For this review, take the finished solid that the model builds, in its own axes (mm). Face numbers are marked on the shaded views. A direction names the side the tool comes from. Give positions to 0.01 mm unless a question says otherwise; leave off trailing zeros. Order: outer loops, then holes, each group sorted by start corner. A loop starts at its lowest first (then second) coordinate and runs counter-clockwise, first axis right, second up. Notation, with made-up numbers: (14, 58) - (40, 58) arc R14 ccw to (40, 62) - close; hole circle Ø7 at (19.5, -23). An arc over 180 degrees is marked (long way). One line per item, written item: value.
Autodesk Inventor part; units mm, degrees
ref_plane "YZ Plane" through (0, 0, 0) normal (1, 0, 0) x (0, 1, 0)
ref_plane "XZ Plane" through (0, 0, 0) normal (0, 1, 0) x (-1, 0, 0)
ref_plane "XY Plane" through (0, 0, 0) normal (0, 0, 1) x (1, 0, 0)
sketch "Sketch1" plane through (0, 0, 0) normal (0, 0, 1) x (1, 0, 0)
  line L0 (0, 0) -> (25, 0)
  line L1 (25, 0) -> (25, 40)
  line L2 (25, 40) -> (0, 40)
  line L3 (0, 40) -> (0, 0)
  dimension "d1" = 25
  dimension "d2" = 40
  dimension "d3" = 25
extrude "Extrusion1" add sketch "Sketch1" against normal blind 30
sketch "Sketch2" plane through (25, 0, 0) normal (1, 0, 0) x (0, 0, -1)
  line L0 (0, 0) -> (30, 0)
  circle A0 centre (15, 6.56) radius 2.46
extrude "Extrusion2" cut sketch "Sketch2" against normal blind 30
sketch "Sketch3" plane through (0, 0, 0) normal (-1, 0, 0) x (0, 0, 1)
  line L0 (0, 0) -> (-30, 0)
  line L1 (-25.05, 0) -> (-4.95, 0)
  line L2 (-4.95, 0) -> (-4.95, 33.12)
  line L3 (-4.95, 33.12) -> (-25.05, 33.12)
  line L4 (-25.05, 33.12) -> (-25.05, 0)
  dimension "d11" = 20.1
extrude "Extrusion3" cut sketch "Sketch3" against normal blind 20
sketch "Sketch4" plane through (0, 0, 0) normal (0, -1, 0) x (1, 0, 0)
  line L0 (20, -4.95) -> (20, -25.05)
  line L1 (20, -15) -> (25, -15)
  line L2 (25, 0) -> (25, -30)
  line L3 (20, -8.025) -> (25, -8.025)
  line L4 (25, -8.025) -> (25, -21.975)
  line L5 (25, -21.975) -> (20, -21.975)
  line L6 (20, -21.975) -> (20, -8.025)
  line L7 (20, -8.025) -> (25, -21.975) construction
  line L8 (25, -8.025) -> (20, -21.975) construction
  line L9 (25, -12.54) -> (25, -17.46)
  point P0 (0, 0)
  point P1 (22.5, -15)
  dimension "d14" = 13.95
extrude "Extrusion4" add sketch "Sketch4" along normal blind 15
sketch "Sketch5" plane through (20, 0, 0) normal (-1, 0, 0) x (0, 0, 1)
  circle A0 centre (-15, 6.56) radius 2.46
  circle A1 centre (-15, 6.56) radius 4.7025
  circle A2 centre (-15, 6.56) radius 2.46
  circle A3 centre (-15, 6.56) radius 2.46
  point P0 (0, 0)
  dimension "d17" = 9.405
extrude "Extrusion5" cut sketch "Sketch5" against normal blind 2.1
sketch "Sketch6" plane through (25, 0, 0) normal (1, 0, 0) x (0, 0, -1)
  circle A0 centre (15, 6.56) radius 4.7025
  line L0 (15, 6.56) -> (15, 23.56)
  circle A1 centre (15, 23.56) radius 2.46
  point P0 (0, 0)
  dimension "d20" = 17
  dimension "d21" = 4.92
extrude "Extrusion6" cut sketch "Sketch6" against normal blind 10 contours A1
sketch "Sketch7" plane through (20, 0, 0) normal (-1, 0, 0) x (0, 0, 1)
  circle A0 centre (-15, 23.56) radius 2.46
  circle A1 centre (-15, 23.56) radius 4.7025
  point P0 (0, 0)
  dimension "d24" = 9.405
extrude "Extrusion7" cut sketch "Sketch7" against normal blind 2.1
sketch "Sketch9" plane through (25, 0, 0) normal (1, 0, 0) x (0, 0, -1)
  circle A0 centre (15, 6.56) radius 2.46
  circle A1 centre (15, 6.56) radius 2.46
  circle A2 centre (15, 23.56) radius 2.46
  circle A3 centre (15, 23.56) radius 2.46
  line L0 (30, 40) -> (30, 0)
  line L1 (30, 0) -> (30, 40)
  line L2 (30, 40) -> (0, 40)
  line L3 (0, 40) -> (0, 0)
  line L4 (0, 0) -> (8.025, 0)
  line L5 (21.975, 0) -> (21.975, -15)
  line L6 (21.975, -15) -> (8.025, -15)
  line L7 (8.025, -15) -> (8.025, 0)
  line L8 (0, 0) -> (8.025, 0)
  line L9 (21.975, 0) -> (30, 0)
extrude "Extrusion8" add sketch "Sketch9" along normal blind 5
sketch "Sketch10" plane through (0, 40, 0) normal (0, 1, 0) x (1, 0, 0)
  line L0 (0, 30) -> (30, 30)
  line L1 (30, 0) -> (0, 0)
  line L2 (0, 30) -> (30, 30)
  line L3 (30, 30) -> (30, 0)
  line L4 (30, 0) -> (0, 0)
  line L5 (0, 0) -> (0, 30)
extrude "Extrusion9" add sketch "Sketch10" along normal blind 30
sketch "Sketch12" plane through (30, 0, 0) normal (1, 0, 0) x (0, 0, -1)
  circle A0 centre (15, 6.56) radius 2.46
  line L0 (15, 6.56) -> (15, 15.06)
  circle A1 centre (15, 15.06) radius 2.525
  point P0 (0, 0)
  dimension "d31" = 8.5
  dimension "d33" = 5.05
extrude "Extrusion10" cut sketch "Sketch12" against normal blind 30 contours A1
sketch "Sketch14" plane through (0, 0, 0) normal (0, 0, 1) x (1, 0, 0)
  line L0 (30, 70) -> (0, 70)
  line L1 (0, 70) -> (0, 85)
  line L2 (-15, 100) -> (-23, 100)
  line L3 (30, 0) -> (30, 70)
  line L4 (30, 113) -> (30, 70)
  arc A0 (0, 85) -> (-15, 100) centre (-15, 85) ccw
  line L5 (30, 105) -> (30, 100)
  line L6 (-23, 128) -> (15, 128)
  line L7 (30, 113) -> (15, 128)
  line L8 (-23, 128) -> (-23, 100)
  point P0 (0, 0)
  point P1 (0, 100)
  dimension "d47" = 30
  dimension "d54" = 15
  dimension "d69" = 28
extrude "Extrusion12" add sketch "Sketch14" against normal blind 30
sketch "Sketch15" plane through (0, 0, -25.05) normal (-1, 0, 0) x (0, 0, 1)
  line L0 (0, 33.12) -> (20.1, 33.12)
  line L1 (20.1, 33.12) -> (20.1, 0)
  line L2 (0, 33.12) -> (20.1, 33.12)
  line L3 (20.1, 33.12) -> (20.1, 31.1)
  line L4 (20.1, 31.1) -> (0, 31.1)
  line L5 (0, 31.1) -> (0, 33.12)
  point P0 (25.05, 0)
  dimension "d57" = 2.02
extrude "Extrusion13" add sketch "Sketch15" against normal blind 20
sketch "Sketch20" plane through (-23, 128, 0) normal (0, 1, 0) x (1, 0, 0)
  line L0 (0, 0) -> (0, 30)
  line L1 (0, 15) -> (0, 9)
  line L2 (0, 21) -> (0, 15)
  line L3 (0, 7.5) -> (0, 22.5)
  line L4 (0, 22.5) -> (2.5, 15)
  line L5 (2.5, 15) -> (0, 7.5)
  point P0 (23, 0)
  dimension "d74" = 6
extrude "Extrusion14" cut sketch "Sketch20" against normal through all
properties part number "24mm_x_30mm"
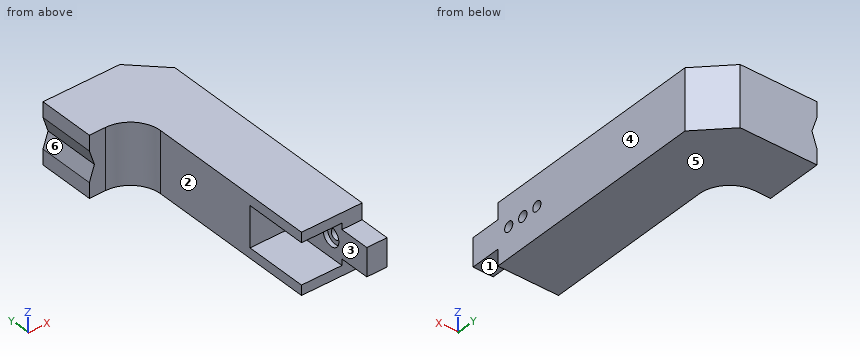
(1) Take a section at A-A (y = 6.56). Write out the cut boundary in (x, z).
Answers below:
outline: (0, -30) - (30, -30) - (30, -17.46) - (22.1, -17.46) - (22.1, -19.7) - (20, -19.7) - (20, -25.05) - (0, -25.05) - close; (0, -4.95) - (20, -4.95) - (20, -10.3) - (22.1, -10.3) - (22.1, -12.54) - (30, -12.54) - (30, 0) - (0, 0) - close
(2) Draft analysis for pull direction X (two halves, no side actions). For the marked faces 4, 5 and 6, state which applies: pulls with the +X half, pulls with the -X half, needs draft (parallel to the pull), parting line crosses it, or undercut.
Answers below:
face 4: pulls with the +X half
face 5: needs draft
face 6: pulls with the -X half
(3) Take a section at B-B (y = 76). Write out the cut boundary in (x, z), then the cut area to 3 significant figures.
Answers below:
outline: (0, -30) - (30, -30) - (30, 0) - (0, 0) - close
area: 900 mm^2
(4) For P1, Ø8, axis at y = 23.56, z = -15, coming from the -X side; P2, Ø10, axis at x = -7, z = -4.5, coming from the -Y side; P3, Ø15, axis at y = 6.56, z = -15, coming from the -X side; P4, Ø4.5, axis at y = 15.06, z = -15, coming from the -X side, all flat-tipped, find the tip position at first contact; note any pin that passes through.
Answers below:
P1: stops at x = 22.1
P2: stops at y = 92.48
P3: stops at x = 20
P4: passes through
(5) Machinability: for the marked faces 1, 2 and 3, which of the approach directions +Z, -Z, +X, -X, +Y, -Y give a long, thin tool a straight path to every point of the face, cutting with its end or side? Answer none if there is none.
Answers below:
face 1: -Z, +X, -X, -Y
face 2: +Z, -Z, -X, -Y
face 3: -X, -Y
(6) Take a section at C-C (x = -10.5). Write out the cut boundary in (y, z), then the cut area to 3 significant figures.
Answers below:
outline: (99.31, -30) - (128, -30) - (128, 0) - (99.31, 0) - close
area: 861 mm^2
(7) Wall thickness on line 1 (Z direction, x = 6, y = 2); line 2 (Y direction, x = 28, z = -15) (3 decimals); line 3 (Z direction, x = 24.25, y = 15.06) (3 decimals): over which ranges is each line inside the solid? List them lowest first. Write a range as from..to.
Answers below:
line 1: z = -30..-25.05, -4.95..0
line 2: y = -15..4.1, 9.02..12.535, 17.585..21.1, 26.02..115
line 3: z = -30..-17.525, -12.475..0
